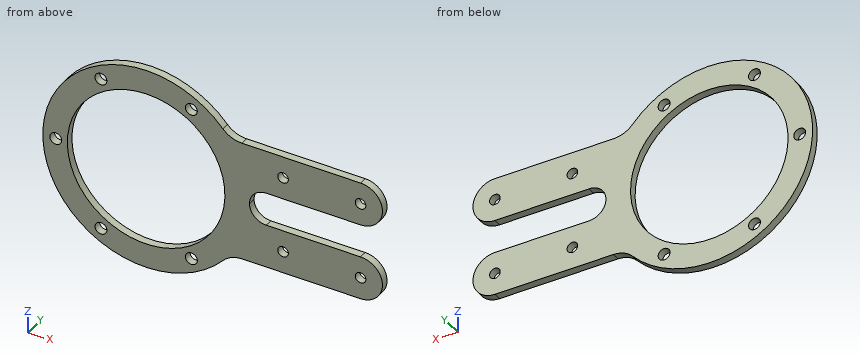
```python
from build123d import *

# Parameters (mm, degrees)
SKETCH1_R           = 40
SKETCH1_R_2         = 30.5
BOSS_EXTRUDE1_DEPTH = 3
BOSS_EXTRUDE2_START = -3
BOSS_EXTRUDE2_DEPTH = 3
SKETCH3_R           = 2.05
CUT_EXTRUDE1_DEPTH  = 108.745069493
SKETCH4_R           = 2.3
CUT_EXTRUDE2_DEPTH  = 108.745069493
CUT_EXTRUDE3_DEPTH  = 108.745069493
FILLET1_R           = 10
FILLET2_R           = 6.5


with BuildPart() as part:
    # Sketch1 → Boss-Extrude1 (new body)
    with BuildSketch(Plane(origin=(0, 0, 0), x_dir=(1, 0, 0), z_dir=(0, 1, 0))):
        with Locations(Location((0, 0, 0), (0, 0, 270))):
            Circle(SKETCH1_R)
        with Locations(Location((0, 0, 0), (0, 0, 270))):
            Circle(SKETCH1_R_2, mode=Mode.SUBTRACT)
    extrude(amount=BOSS_EXTRUDE1_DEPTH)

    # Sketch2 → Boss-Extrude2 (add)
    with BuildSketch(Plane(origin=(0, 3, 0), x_dir=(1, 0, 0), z_dir=(0, 1, 0)).offset(BOSS_EXTRUDE2_START)):
        with BuildLine():
            Line((100, 6.5), (39.468341744, 6.5))
            ThreePointArc((39.468341744, 6.5), (36.910699238, 15.414288235), (32.368966619, 23.5))
            Line((32.368966619, 23.5), (100, 23.5))
            Line((100, 23.5), (100, 6.5))
        make_face()
        with BuildLine():
            Line((39.468341744, -6.5), (100, -6.5))
            Line((100, -6.5), (100, -23.5))
            Line((100, -23.5), (32.368966619, -23.5))
            ThreePointArc((32.368966619, -23.5), (36.910699238, -15.414288235), (39.468341744, -6.5))
        make_face()
    extrude(amount=BOSS_EXTRUDE2_DEPTH)

    # Sketch3 → Cut-Extrude1 (cut, through all)
    with BuildSketch(Plane(origin=(0, 3, 0), x_dir=(1, 0, 0), z_dir=(0, 1, 0))):
        with Locations(Location((53, 15, 0), (0, 0, 270))):
            Circle(SKETCH3_R)
        with Locations(Location((83, 15, 0), (0, 0, 270))):
            Circle(SKETCH3_R)
        with Locations(Location((53, -15, 0), (0, 0, 270))):
            Circle(SKETCH3_R)
        with Locations(Location((83, -15, 0), (0, 0, 270))):
            Circle(SKETCH3_R)
    extrude(amount=-CUT_EXTRUDE1_DEPTH, mode=Mode.SUBTRACT)

    # Sketch4 → Cut-Extrude2 (cut, through all)
    with BuildSketch(Plane(origin=(0, 3, 0), x_dir=(1, 0, 0), z_dir=(0, 1, 0))):
        with Locations(Location((-17.5, 30.310889132, 0), (0, 0, 270))):
            Circle(SKETCH4_R)
        with Locations(Location((17.5, 30.310889132, 0), (0, 0, 270))):
            Circle(SKETCH4_R)
        with Locations(Location((17.5, -30.310889132, 0), (0, 0, 270))):
            Circle(SKETCH4_R)
        with Locations(Location((-17.5, -30.310889132, 0), (0, 0, 270))):
            Circle(SKETCH4_R)
        with Locations(Location((-35, 0, 0), (0, 0, 270))):
            Circle(SKETCH4_R)
    extrude(amount=-CUT_EXTRUDE2_DEPTH, mode=Mode.SUBTRACT)

    # Sketch6 → Cut-Extrude3 (cut, through all)
    with BuildSketch(Plane(origin=(0, 3, 0), x_dir=(1, 0, 0), z_dir=(0, 1, 0))):
        with BuildLine():
            Line((100, 23.5), (83, 23.5))
            ThreePointArc((83, 23.5), (91.5, 15), (83, 6.5))
            Line((83, 6.5), (100, 6.5))
            Line((100, 6.5), (100, 23.5))
        make_face()
        with BuildLine():
            Line((100, -6.5), (83, -6.5))
            ThreePointArc((83, -6.5), (91.5, -15), (83, -23.5))
            Line((83, -23.5), (100, -23.5))
            Line((100, -23.5), (100, -6.5))
        make_face()
    extrude(amount=-CUT_EXTRUDE3_DEPTH, mode=Mode.SUBTRACT)

    # Fillet1
    fillet1_edges = [part.edges().sort_by_distance(p)[0] for p in [
        (32.368966619, 1.5, -23.5),
        (32.368966619, 1.5, 23.5),
    ]]
    fillet(fillet1_edges, radius=FILLET1_R)

    # Fillet2
    fillet2_edges = [part.edges().sort_by_distance(p)[0] for p in [
        (39.468341744, 1.5, 6.5),
        (39.468341744, 1.5, -6.5),
    ]]
    fillet(fillet2_edges, radius=FILLET2_R - 0.0001)  # a hair under: the kernel refuses the full size


solid = part.part
```
Can you work these out from the model? Positions are in its coordinate system, mm. Round coordinates to 2 decimals unless told otherwise and drop trailing zeros. Loops run counter-clockwise (first coordinate to the right, second up) from the corner with the lowest first, then second, coordinate; pieces in that order, holes last. Notation, with made-up numbers: M 26,38 L 58,38 A30 cw 58,70 Z; hole C 19,79.5 d7. An arc over 180 degrees is marked long. Answer as a JSON object with one key per item and string values. Group by question number.
Q1. Will these pins go through, and if not, where does the flat tip stop? pin 1 (3 mm diameter, centred on x = 26, z = -18.5, fed in from -Y); pin 2 (1.5 mm diameter, centred on y = 1.5, z = 19.5, fed in from +X); pin 3 (1.5 mm diameter, centred on x = 55.5, y = 2, fed in from -Z); pin 4 (0.9 mm diameter, centred on x = 50.5, y = 1.5, fed in from +Z).
Q2. Imagine slicing it at C-C, the plane x = 53. Please give me the cut outline in (y, z).
Q3. Imagine slicing it at A-A, the plane x = 70.5. Please give me the cut outline in (y, z), then the cut area to 3 significant figures.
Q4. Imagine slicing it at D-D, the plane z = 15. Please give me the cut outline in (x, y).
Q5. Imagine slicing it at B-B, the plane y = 2.4. Count the separate pieces of the cut face and the enclosed holes in it, then the cut area to 3 significant figures.
Q6. Please list where these lines run through material, in increasing order: L1, parallel to X at y = 1.75, z = 15; L2, parallel to X at y = 0.2, z = 1.5; L3, parallel to X at y = 1.6, z = 16.
Findings:
{
 "1": {"pin 1": "stops at y = 0", "pin 2": "stops at x = 90.63", "pin 3": "stops at z = -23.5", "pin 4": "stops at z = 23.5"},
 "2": {"outline": "M 0,-23.5 L 3,-23.5 L 3,-17.05 L 0,-17.05 Z; M 0,-12.95 L 3,-12.95 L 3,-6.5 L 0,-6.5 Z; M 0,6.5 L 3,6.5 L 3,12.95 L 0,12.95 Z; M 0,17.05 L 3,17.05 L 3,23.5 L 0,23.5 Z"},
 "3": {"outline": "M 0,-23.5 L 3,-23.5 L 3,-6.5 L 0,-6.5 Z; M 0,6.5 L 3,6.5 L 3,23.5 L 0,23.5 Z", "area": "102 mm2"},
 "4": {"outline": "M -37.08,0 L -26.56,0 L -26.56,3 L -37.08,3 Z; M 26.56,0 L 50.95,0 L 50.95,3 L 26.56,3 Z; M 55.05,0 L 80.95,0 L 80.95,3 L 55.05,3 Z; M 85.05,0 L 91.5,0 L 91.5,3 L 85.05,3 Z"},
 "5": {"separate pieces": "1", "enclosed holes": "10", "area": "3,800 mm2"},
 "6": {"L1": "x = -37.08 to -26.56, 26.56 to 50.95, 55.05 to 80.95, 85.05 to 91.5", "L2": "x = -39.97 to -36.74, -33.26 to -30.46, 30.46 to 40.18", "L3": "x = -36.66 to -25.97, 25.97 to 51.21, 54.79 to 81.21, 84.79 to 91.44"}
}
